Autodesk Inventor part; units mm, degrees
ref_plane "YZ Plane" through (0, 0, 0) normal (1, 0, 0) x (0, 1, 0)
ref_plane "XZ Plane" through (0, 0, 0) normal (0, 1, 0) x (-1, 0, 0)
ref_plane "XY Plane" through (0, 0, 0) normal (0, 0, 1) x (1, 0, 0)
sketch "Sketch1" plane through (0, 0, 0) normal (0, 1, 0) x (-1, 0, 0)
  line L0 (0, 0) -> (-50, 0)
  line L1 (-50, 0) -> (-50, -54.112)
  line L2 (-50, -54.112) -> (0, -54.112)
  line L3 (0, -54.112) -> (0, 0)
  dimension "d0" = 50
  dimension "d1" = 54.112
extrude "Extrusion1" add sketch "Sketch1" along normal blind 4
sketch "Sketch2" plane through (50, 0, -54.112) normal (0, 0, -1) x (-1, 0, 0)
  line L0 (50, 0) -> (42, 0)
  line L1 (0, 0) -> (50, 0)
  line L2 (42, 0) -> (42, -4)
  circle A0 centre (42, -4) radius 4
  circle A1 centre (42, -4) radius 8
  line L3 (50, -4) -> (50, 0)
  line L4 (34, -4) -> (34, 0)
  line L5 (34, 0) -> (35.0718, 0)
  line L6 (50, 0) -> (48.9282, 0)
  dimension "d4" = 8
  dimension "d6" = 4
  dimension "d7" = 16
extrude "Extrusion2" add sketch "Sketch2" against normal blind 54.112 contours L3 A1 L0 | A1 L1 L0 | A1 L4 L1 picked at (48.5892, -4.6382)
sketch "Sketch4" plane through (0, 0, 0) normal (0, -1, 0) x (1, 0, 0)
  line L0 (50, -54.112) -> (16, -54.112)
  line L1 (16, -54.112) -> (26, -54.112)
  line L2 (26, -54.112) -> (26, -44.112)
  line L3 (0, 0) -> (50, 0)
  line L4 (26, 0) -> (16, 0)
  line L5 (26, 0) -> (26, -10)
  line L6 (26, -10) -> (46, -10)
  line L7 (26, -44.112) -> (46, -44.112)
  circle A0 centre (46, -44.112) radius 2.5
  circle A1 centre (46, -10) radius 2.5
  circle A2 centre (26, -10) radius 2.5
  circle A3 centre (26, -44.112) radius 2.5
  dimension "d10" = 10
  dimension "d11" = 10
  dimension "d12" = 10
  dimension "d13" = 10
  dimension "d14" = 20
  dimension "d15" = 20
  dimension "d16" = 5
  dimension "d17" = 5
  dimension "d18" = 5
  dimension "d19" = 5
extrude "Extrusion3" cut sketch "Sketch4" against normal blind 54.112
sketch "Sketch5" plane through (0, 4, -54.112) normal (-1, 0, 0) x (0, 0, 1)
  line L0 (0, 0) -> (54.112, 0)
  line L1 (0, 0) -> (54.112, 0)
  line L2 (54.112, 0) -> (54.112, 20)
  line L3 (54.112, 20) -> (0, 20)
  line L4 (0, 20) -> (0, 0)
  point P0 (54.112, -4)
  dimension "d22" = 20
extrude "Extrusion4" add sketch "Sketch5" along normal blind 5
sketch "Sketch6" plane through (50, 0, 0) normal (0, 0, 1) x (1, 0, 0)
  line L0 (-50, 4) -> (-55, 4)
  line L1 (-50, -4) -> (-50, 4)
  line L2 (-55, 4) -> (-50, -4)
  line L3 (-50, -4) -> (-50, 4)
  line L4 (-50, 4) -> (-55, 4)
  point P0 (-50, 0)
extrude "Extrusion5" add sketch "Sketch6" against normal up to surface (54.112 mm away)
sketch "Sketch7" plane through (-5, 4, -54.112) normal (-1, 0, 0) x (0, 0, 1)
  line L0 (0, 0) -> (27.056, 0)
  line L1 (0, 20) -> (0, 0)
  line L2 (0, 0) -> (10, 0)
  line L3 (10, 0) -> (10, 10)
  line L4 (0, 0) -> (54.112, 0)
  line L5 (54.112, 0) -> (44.112, 0)
  line L6 (44.112, 0) -> (44.112, 10)
  circle A0 centre (10, 10) radius 2.5
  circle A1 centre (44.112, 10) radius 2.5
  point P0 (54.112, -4)
  dimension "d45" = 10
  dimension "d46" = 10
  dimension "d47" = 10
  dimension "d48" = 5
  dimension "d49" = 5
extrude "Extrusion6" cut sketch "Sketch7" against normal blind 10
sketch "Sketch8" plane through (50, 0, 0) normal (1, 0, 0) x (0, 0, -1)
  line L0 (54.112, 4) -> (0, 4)
  line L1 (0, 0) -> (54.112, 0)
  line L2 (0, 4) -> (54.112, 4)
  line L3 (54.112, 4) -> (54.112, 0)
  line L4 (54.112, 0) -> (0, 0)
  line L5 (0, 0) -> (0, 4)
extrude "Extrusion7" add sketch "Sketch8" along normal blind 7.5
sketch "Sketch9" plane through (16, -4, -54.112) normal (1, 0, 0) x (0, 0, -1)
  line L0 (0, 0) -> (-54.112, 0)
  line L1 (-54.112, 0) -> (-27.056, 0)
  circle A0 centre (-27.056, 0) radius 2
  point P0 (-54.112, 4)
  dimension "d33" = 4
hole "Hole1" at (16, -4, -27.056) direction (-1, 0, 0) diameter 4 end up to surface
thread "Thread2"
properties part number "4x2020_subaxis" material "PET Plastic"
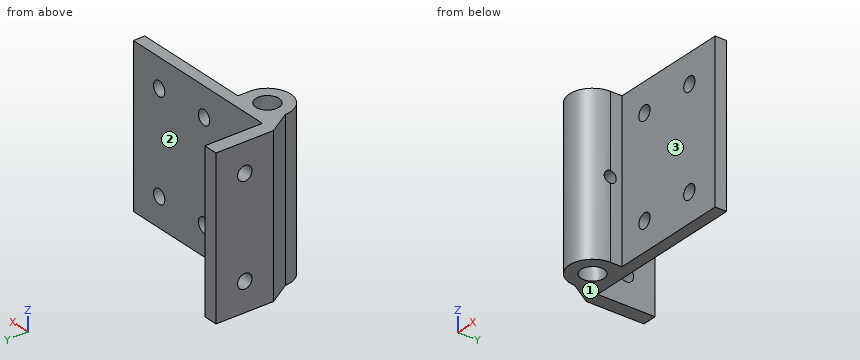
The listing builds one solid part. Answer for the finished solid, in the listing's coordinates (mm). Face numbers are marked on the shaded views. A direction names the side the tool comes from. Give positions to 0.01 mm unless a question says otherwise; leave off trailing zeros. Write each loop counter-clockwise with the first axis right and the second up, starting at its lowest first coordinate (ties: lowest second). Pieces come first, ordered by that corner, then holes. Notation, with made-up numbers: (22, 53.25) -> (26, 53.25) arc R28 ccw to (26, 74.25) -> close; hole circle Ø9 at (4.5, -38.5). An arc over 180 degrees is marked (long way). One line per question, with ' | ' between items. Start each with the question number.
1. Section D-D (y = 14) is taken. Determine the outline of the cut face in (x, z), plus the area to 3 significant figures.
2. Section C-C (x = 8) is taken. Determine the outline of the cut face in (y, z).
3. Find the intervals of material crossed by probe 1 along Z at (x, y) = (26, 2.35); probe 2 along X at (y, z) = (2.95, -10); probe 3 along X at (y, z) = (3, -10) (3 decimals), in increasing order.
4. Section A-A (z = -10) is taken. Determine the outline of the cut face in (x, y), plus the area to 3 significant figures.
5. Given pin 1 Ø10 at (x, z) = (50.5, -37.5) entering from -Y; pin 2 Ø12 at (x, y) = (10, 12.5) entering from -Z (3 decimals); pin 3 Ø1 at (y, z) = (-8, -7) entering from +X; pin 4 Ø2 at (x, z) = (17, -22) entering from +Y, each flat-ended and moving along its own axis, determine where each tip first touches the part or whether it passes through.
6. Section B-B (x = 26) is taken. Determine the outline of the cut face in (y, z), plus the area to 3 significant figures.
7. For the marked faces 1, 2 and 3, determine the directions among +Z, -Z, +X, -X, +Y, -Y from which every point of the face is accessible in a straight line to the end or side of a thin tool.
Response values:
1) outline: (-5, -54.11) -> (0, -54.11) -> (0, -46.61) -> (-5, -46.61) -> close; (-5, -41.61) -> (0, -41.61) -> (0, -12.5) -> (-5, -12.5) -> close; (-5, -7.5) -> (0, -7.5) -> (0, 0) -> (-5, 0) -> close | area: 221 mm2
2) outline: (-12, -54.11) -> (-8, -54.11) -> (-8, 0) -> (-12, 0) -> close; (0, -54.11) -> (4, -54.11) -> (4, 0) -> (0, 0) -> close
3) probe 1: -54.11 to -46.61, -41.61 to -12.5, -7.5 to 0 | probe 2: -4.34 to 23.5, 28.5 to 43.5, 48.5 to 57.5 | probe 3: -4.375 to 23.5, 28.5 to 43.5, 48.5 to 57.5
4) outline: (-5, 4) -> (0, -4) arc R8 ccw to (16, -4) -> (16, 0) -> (23.5, 0) -> (23.5, 4) -> (0, 4) -> (0, 11.5) -> (-5, 11.5) -> close; (-5, 16.5) -> (0, 16.5) -> (0, 24) -> (-5, 24) -> close; (28.5, 0) -> (43.5, 0) -> (43.5, 4) -> (28.5, 4) -> close; (48.5, 0) -> (57.5, 0) -> (57.5, 4) -> (48.5, 4) -> close; hole circle Ø8 at (8, -4) | area: 399 mm2
5) pin 1: y = 0 | pin 2: through | pin 3: x = 15.19 | pin 4: y = 4
6) outline: (0, -54.11) -> (4, -54.11) -> (4, -46.61) -> (0, -46.61) -> close; (0, -41.61) -> (4, -41.61) -> (4, -12.5) -> (0, -12.5) -> close; (0, -7.5) -> (4, -7.5) -> (4, 0) -> (0, 0) -> close | area: 176 mm2
7) face 1: -Z, +X, -X, +Y, -Y | face 2: +Z, -Z, +X, +Y | face 3: +Z, -Z, +X, -Y
